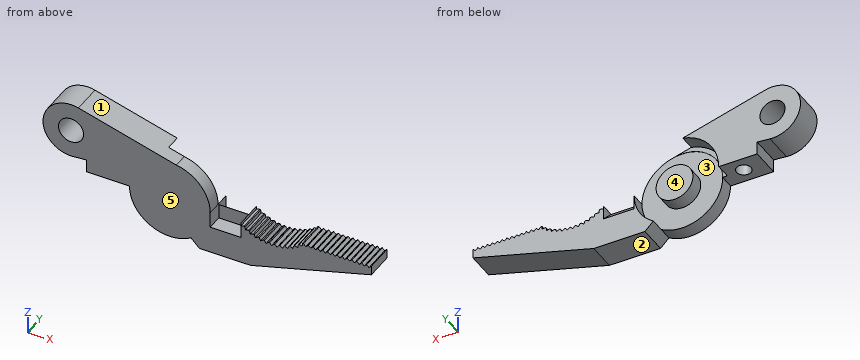
```python
from build123d import *

# Parameters (mm, degrees)
SKETCH1_R                        = 6.5405
SKETCH1_R_2                      = 2.9845
BOSS_EXTRUDE1_DEPTH              = 4.826
SKETCH2_R                        = 2.032
BOSS_EXTRUDE2_DEPTH              = 4.826
F_42_0_0935_DIAMETER_HOLE1_D     = 2.3749
F_42_0_0935_DIAMETER_HOLE1_DEPTH = 2.032
F_42_0_0935_DIAMETER_HOLE1_TIP   = 0.713491942
BOSS_EXTRUDE3_DEPTH              = 4.826
CUT_EXTRUDE1_DEPTH               = 2.50825
CUT_EXTRUDE2_DEPTH               = 5.826
LPATTERN1_COUNT                  = 14
LPATTERN1_PITCH                  = 0.7874
CUT_EXTRUDE3_DEPTH               = 5.826
CIRPATTERN1_COUNT                = 13
CIRPATTERN1_ANGLE                = 76.5
SKETCH13_W                       = 4.971607039
SKETCH13_H                       = 2.54
CUT_EXTRUDE5_DEPTH               = 2.50825
BOSS_EXTRUDE4_REACH              = 28.099
SKETCH15_W                       = 4.971607039
SKETCH15_H                       = 2.54
CUT_EXTRUDE6_DEPTH               = 2.50825
SKETCH16_R                       = 6.5405
CUT_EXTRUDE7_DEPTH               = 2.54
SKETCH18_R                       = 2.9845
BOSS_EXTRUDE5_DEPTH              = 4.572
CUT_EXTRUDE8_DEPTH               = 0.254
CUT_EXTRUDE9_REACH               = 34.057


with BuildPart() as part:
    # Sketch1 → Boss-Extrude1 (new body)
    with BuildSketch(Plane(origin=(0, 0, 0), x_dir=(1, 0, 0), z_dir=(0, 1, 0))):
        Circle(SKETCH1_R)
        Circle(SKETCH1_R_2, mode=Mode.SUBTRACT)
    extrude(amount=BOSS_EXTRUDE1_DEPTH)

    # Sketch2 → Boss-Extrude2 (add)
    with BuildSketch(Plane(origin=(0, 0, 0), x_dir=(1, 0, 0), z_dir=(0, 1, 0))):
        with BuildLine():
            Line((-6.5405, 0), (-13.5255, 0))
            Line((-13.5255, 0), (-13.5255, -2.088510966))
            Line((-13.5255, -2.088510966), (-15.606063552, -1.906485242))
            ThreePointArc((-15.606063552, -1.906485242), (-20.526278057, -6.842542927), (-14.798031619, -10.81247605))
            Line((-14.798031619, -10.81247605), (1.058408056, -6.454294124))
            ThreePointArc((1.058408056, -6.454294124), (-4.234124606, -4.985010438), (-6.5405, 0))
        make_face()
        with Locations((-16.002, -6.432059555)):
            Circle(SKETCH2_R, mode=Mode.SUBTRACT)
    extrude(amount=BOSS_EXTRUDE2_DEPTH)

    # #42 (0.0935) Diameter Hole1
    with Locations(Plane(origin=(0, 0, 0), x_dir=(-1, 0, 0), z_dir=(0, 0, -1))):
        with Locations((10.033, 2.413)):
            Hole(F_42_0_0935_DIAMETER_HOLE1_D / 2, depth=F_42_0_0935_DIAMETER_HOLE1_DEPTH)
            with Locations((0, 0, -(F_42_0_0935_DIAMETER_HOLE1_DEPTH + F_42_0_0935_DIAMETER_HOLE1_TIP / 2))):  # 118° drill point
                Cone(0, F_42_0_0935_DIAMETER_HOLE1_D / 2, F_42_0_0935_DIAMETER_HOLE1_TIP, mode=Mode.SUBTRACT)

    # Sketch8 → Boss-Extrude3 (add)
    with BuildSketch(Plane(origin=(0, 0, 0), x_dir=(1, 0, 0), z_dir=(0, 1, 0))):
        with BuildLine():
            Line((13.081, 6.9342), (32.639, 1.524))
            Line((32.639, 1.524), (32.639, 0))
            Line((32.639, 0), (21.463, 0))
            ThreePointArc((21.463, 0), (16.51, 1.829301337), (11.557, 0))
            Line((11.557, 0), (6.5405, 0))
            ThreePointArc((6.5405, 0), (5.709882431, 3.189887596), (3.429, 5.569569036))
            Line((3.429, 5.569569036), (4.793630964, 6.9342))
            Line((4.793630964, 6.9342), (13.081, 6.9342))
        make_face()
    extrude(amount=BOSS_EXTRUDE3_DEPTH)

    # Sketch9 → Cut-Extrude1 (cut)
    with BuildSketch(Plane(origin=(0, 4.826, 0), x_dir=(1, 0, 0), z_dir=(0, 1, 0))):
        with BuildLine():
            Line((-6.5405, 0), (-7.3025, 0))
            ThreePointArc((-7.3025, 0), (-5.662092509, -4.611639044), (-1.477860583, -7.151393874))
            Line((-1.477860583, -7.151393874), (1.058408056, -6.454294124))
            ThreePointArc((1.058408056, -6.454294124), (-4.234124606, -4.985010438), (-6.5405, 0))
        make_face()
    extrude(amount=-CUT_EXTRUDE1_DEPTH, mode=Mode.SUBTRACT)

    # Sketch10 → Cut-Extrude2 (cut, through all)
    with BuildSketch(Plane(origin=(0, 4.826, 0), x_dir=(1, 0, 0), z_dir=(0, 1, 0))):
        Polygon((32.639, 0), (32.258, 0.381), (31.877, 0), align=None)
    cut_extrude2 = extrude(amount=-CUT_EXTRUDE2_DEPTH, mode=Mode.SUBTRACT)

    # LPattern1: Cut-Extrude2 ×14
    with Locations(*[(-i * LPATTERN1_PITCH, 0, 0) for i in range(1, LPATTERN1_COUNT)]):
        add(cut_extrude2, mode=Mode.SUBTRACT)

    # Sketch11 → Cut-Extrude3 (cut, through all)
    with BuildSketch(Plane(origin=(0, 4.826, 0), x_dir=(1, 0, 0), z_dir=(0, 1, 0))):
        with BuildLine():
            Line((21.463, 0), (21.438001029, 0.512539145))
            Line((21.438001029, 0.512539145), (20.934572554, 0.413135452))
            ThreePointArc((20.934572554, 0.413135452), (21.203334313, 0.212384964), (21.463, 0))
        make_face()
    cut_extrude3 = extrude(amount=-CUT_EXTRUDE3_DEPTH, mode=Mode.SUBTRACT)

    # CirPattern1: Cut-Extrude3 ×13 about axis
    cirpattern1_axis = Axis((16.51, 0, 5.790698663), (0, 1, 0))
    for i in range(1, CIRPATTERN1_COUNT):
        add(cut_extrude3.rotate(cirpattern1_axis, i * CIRPATTERN1_ANGLE / (CIRPATTERN1_COUNT - 1)), mode=Mode.SUBTRACT)

    # Sketch13 → Cut-Extrude5 (cut)
    with BuildSketch(Plane(origin=(0, 4.826, 0), x_dir=(1, 0, 0), z_dir=(0, 1, 0))):
        with Locations((9.02630352, 1.27)):
            Rectangle(SKETCH13_W, SKETCH13_H)
    extrude(amount=-CUT_EXTRUDE5_DEPTH, mode=Mode.SUBTRACT)

    # Sketch14 → Boss-Extrude4 (add, up to next)
    with BuildSketch(Plane(origin=(6.5405, 0, 0), x_dir=(0, 0, -1), z_dir=(1, 0, 0)), mode=Mode.PRIVATE) as boss_extrude4_sk1:
        Polygon((0, 2.31775), (2.54, 4.826), (2.54, 2.31775), align=None)
    boss_extrude4_tool1 = extrude(boss_extrude4_sk1.sketch, amount=BOSS_EXTRUDE4_REACH, mode=Mode.PRIVATE) - part.part
    add(boss_extrude4_tool1.solids().sort_by_distance((6.5405, 3.153833, -1.693333))[0])

    # Sketch15 → Cut-Extrude6 (cut)
    with BuildSketch(Plane.XZ):
        with Locations((9.02630352, -1.27)):
            Rectangle(SKETCH15_W, SKETCH15_H)
    extrude(amount=-CUT_EXTRUDE6_DEPTH, mode=Mode.SUBTRACT)

    # Sketch16 → Cut-Extrude7 (cut)
    with BuildSketch(Plane(origin=(0, 4.826, 0), x_dir=(1, 0, 0), z_dir=(0, 1, 0))):
        Circle(SKETCH16_R)
    extrude(amount=-CUT_EXTRUDE7_DEPTH, mode=Mode.SUBTRACT)

    # Sketch18 → Boss-Extrude5 (add)
    with BuildSketch(Plane(origin=(0, 0, 0), x_dir=(1, 0, 0), z_dir=(0, 1, 0))):
        Circle(SKETCH18_R)
    extrude(amount=BOSS_EXTRUDE5_DEPTH)

    # Sketch19 → Cut-Extrude8 (cut)
    with BuildSketch(Plane(origin=(0, 4.826, 0), x_dir=(1, 0, 0), z_dir=(0, 1, 0))):
        with BuildLine():
            Line((6.5405, 0), (6.5405, 2.54))
            Line((6.5405, 2.54), (11.512107039, 2.54))
            Line((11.512107039, 2.54), (11.512107039, 0))
            Line((11.512107039, 0), (11.531340148, 0.472602949))
            Line((11.531340148, 0.472602949), (12.03555369, 0.377261309))
            ThreePointArc((12.03555369, 0.377261309), (12.10743347, 0.428771407), (12.179906178, 0.479443879))
            Line((12.179906178, 0.479443879), (12.257573507, 0.986680619))
            Line((12.257573507, 0.986680619), (12.748082937, 0.835943022))
            ThreePointArc((12.748082937, 0.835943022), (12.825237685, 0.879153411), (12.90288869, 0.921465519))
            Line((12.90288869, 0.921465519), (13.036396947, 1.416941925))
            Line((13.036396947, 1.416941925), (13.507136098, 1.212672553))
            ThreePointArc((13.507136098, 1.212672553), (13.588611636, 1.247048848), (13.67048062, 1.280477314))
            Line((13.67048062, 1.280477314), (13.8581787, 1.758065792))
            Line((13.8581787, 1.758065792), (14.303325905, 1.502790861))
            ThreePointArc((14.303325905, 1.502790861), (14.388114618, 1.527907928), (14.473189102, 1.55203934))
            Line((14.473189102, 1.55203934), (14.712755728, 2.005833517))
            Line((14.712755728, 2.005833517), (15.126805817, 1.702710031))
            ThreePointArc((15.126805817, 1.702710031), (15.213859118, 1.718257244), (15.301086979, 1.732793167))
            Line((15.301086979, 1.732793167), (15.589559413, 2.157180937))
            Line((15.589559413, 2.157180937), (15.967391797, 1.809957647))
            ThreePointArc((15.967391797, 1.809957647), (16.05563309, 1.815742734), (16.143935576, 1.8205034))
            Line((16.143935576, 1.8205034), (16.477746256, 2.210236326))
            Line((16.477746256, 2.210236326), (16.814688254, 1.82320737))
            ThreePointArc((16.814688254, 1.82320737), (16.903026252, 1.819158785), (16.991311318, 1.81408532))
            Line((16.991311318, 1.81408532), (17.366331983, 2.164343546))
            Line((17.366331983, 2.164343546), (17.658216609, 1.742295339))
            ThreePointArc((17.658216609, 1.742295339), (17.745558829, 1.728463151), (17.832734648, 1.713618299))
            Line((17.832734648, 1.713618299), (18.244327388, 2.020070154))
            Line((18.244327388, 2.020070154), (18.487544881, 1.568222199))
            ThreePointArc((18.487544881, 1.568222199), (18.572811157, 1.544777473), (18.657799617, 1.52034482))
            Line((18.657799617, 1.52034482), (19.100874234, 1.779200392))
            Line((19.100874234, 1.779200392), (19.292416706, 1.303140726))
            ThreePointArc((19.292416706, 1.303140726), (19.374552542, 1.270373405), (19.456302586, 1.236655112))
            Line((19.456302586, 1.236655112), (19.925379542, 1.444713114))
            Line((19.925379542, 1.444713114), (20.062878172, 0.950329204))
            ThreePointArc((20.062878172, 0.950329204), (20.140867788, 0.908644522), (20.218368406, 0.866057587))
            Line((20.218368406, 0.866057587), (20.707646593, 1.02074495))
            Line((20.707646593, 1.02074495), (20.789400924, 0.514150878))
            ThreePointArc((20.789400924, 0.514150878), (20.862279817, 0.464064354), (20.934572554, 0.413135452))
            Line((20.934572554, 0.413135452), (21.438001029, 0.512539145))
            Line((21.438001029, 0.512539145), (21.463, 0))
            Line((21.463, 0), (21.6408, 0))
            Line((21.6408, 0), (22.0218, 0.381))
            Line((22.0218, 0.381), (22.4028, 0))
            Line((22.4028, 0), (22.4282, 0))
            Line((22.4282, 0), (22.8092, 0.381))
            Line((22.8092, 0.381), (23.1902, 0))
            Line((23.1902, 0), (23.2156, 0))
            Line((23.2156, 0), (23.5966, 0.381))
            Line((23.5966, 0.381), (23.9776, 0))
            Line((23.9776, 0), (24.003, 0))
            Line((24.003, 0), (24.384, 0.381))
            Line((24.384, 0.381), (24.765, 0))
            Line((24.765, 0), (24.7904, 0))
            Line((24.7904, 0), (25.1714, 0.381))
            Line((25.1714, 0.381), (25.5524, 0))
            Line((25.5524, 0), (25.5778, 0))
            Line((25.5778, 0), (25.9588, 0.381))
            Line((25.9588, 0.381), (26.3398, 0))
            Line((26.3398, 0), (26.3652, 0))
            Line((26.3652, 0), (26.7462, 0.381))
            Line((26.7462, 0.381), (27.1272, 0))
            Line((27.1272, 0), (27.1526, 0))
            Line((27.1526, 0), (27.5336, 0.381))
            Line((27.5336, 0.381), (27.9146, 0))
            Line((27.9146, 0), (27.94, 0))
            Line((27.94, 0), (28.321, 0.381))
            Line((28.321, 0.381), (28.702, 0))
            Line((28.702, 0), (28.7274, 0))
            Line((28.7274, 0), (29.1084, 0.381))
            Line((29.1084, 0.381), (29.4894, 0))
            Line((29.4894, 0), (29.5148, 0))
            Line((29.5148, 0), (29.8958, 0.381))
            Line((29.8958, 0.381), (30.2768, 0))
            Line((30.2768, 0), (30.3022, 0))
            Line((30.3022, 0), (30.6832, 0.381))
            Line((30.6832, 0.381), (31.0642, 0))
            Line((31.0642, 0), (31.0896, 0))
            Line((31.0896, 0), (31.4706, 0.381))
            Line((31.4706, 0.381), (31.8516, 0))
            Line((31.8516, 0), (31.877, 0))
            Line((31.877, 0), (32.258, 0.381))
            Line((32.258, 0.381), (32.639, 0))
            Line((32.639, 0), (32.639, 1.524))
            Line((32.639, 1.524), (13.081, 6.9342))
            Line((13.081, 6.9342), (4.793630964, 6.9342))
            Line((4.793630964, 6.9342), (3.429, 5.569569036))
            ThreePointArc((3.429, 5.569569036), (5.709882431, 3.189887596), (6.5405, 0))
        make_face()
    extrude(amount=-CUT_EXTRUDE8_DEPTH, mode=Mode.SUBTRACT)

    # Sketch20 → Cut-Extrude9 (cut, up to next)
    with BuildSketch(Plane(origin=(11.512107039, 0, 0), x_dir=(0, 0, -1), z_dir=(1, 0, 0)), mode=Mode.PRIVATE) as cut_extrude9_sk1:
        Polygon((2.54, 4.826), (2.28278481, 4.572), (2.54, 4.572), align=None)
    cut_extrude9_tool1 = extrude(cut_extrude9_sk1.sketch, amount=-CUT_EXTRUDE9_REACH, mode=Mode.PRIVATE) & part.part
    add(cut_extrude9_tool1.solids().sort_by_distance((11.512107, 4.656667, -2.454262))[0], mode=Mode.SUBTRACT)


solid = part.part
```
The model under review builds one solid part; all positions refer to its coordinate system, in mm. Face numbers are marked on the shaded views. A direction names the side the tool comes from. Give positions to 0.01 mm unless a question says otherwise; leave off trailing zeros. Use CSV: the item, a comma, the result in double quotes. Start each with the question number.
Q1. Clearance check with flat-ended pins moving along their axes: pin 1 Ø1 at (x, z) = (24.5, 0) entering from -Y; pin 2 Ø1.7 at (y, z) = (2.5, 1.5) entering from -X; pin 3 Ø1.4 at (x, y) = (-9.5, 2.5) entering from -Z; pin 4 Ø0.8 at (y, z) = (1, -1) entering from -X. State where each tip first meets the part, or that it passes through.
Q2. We need section B-B, the plane y = 4.1. State how many separate pieces and enclosed holes the cut face has, and give its area (3 significant figures).
Q3. To check wall thickness, follow line 1 along Y through (x, z) = (27, -2); line 2 along Y through (x, z) = (-9, 2); line 3 along X through (y, z) = (3.4, 6). State the ranges of each line that lie inside material, in increasing order. Write a range as [from, to].
Q4. The part is to be moulded in two halves that separate along X. For the marked faces 1, 2 and 3, say which applies: +X half, -X half, draft (parallel to the pull), parting line (faces both ways), or undercut.
Q5. Tool access review of the marked faces 4 and 5: name each direction out of +Z, -Z, +X, -X, +Y, -Y from which nothing blocks a thin tool from reaching the whole face with its end or side.
Outcome:
1,pin 1,"stops at y = 0"
1,pin 2,"stops at x = -18"
1,pin 3,"stops at z = 0"
1,pin 4,"stops at x = -6.51"
2,separate pieces,"3"
2,enclosed holes,"1"
2,area,"256 mm^2"
3,line 1,"y = [0, 4.57]"
3,line 2,"y = [0, 1.83], [3, 4.83]"
3,line 3,"x = [-20.52, -17.99], [-14.02, -4.16]"
4,face 1,"+X half"
4,face 2,"draft"
4,face 3,"undercut"
5,face 4,"-Z, +X, +Y"
5,face 5,"+Z, -Z, +X, -X, -Y"
